Design review of the part shown in the three views and the two pictorial views. Dimensions are in mm from the part's minimum x, y and z. A direction names the side the tool comes from. Coordinates: 2 decimals unless noted, no trailing zeros. Loops run counter-clockwise (first coordinate to the right, second up) from the corner with the lowest first, then second, coordinate; pieces in that order, holes last. Notation, with made-up numbers: (12, 78.5) - (24, 78.5) arc R19 ccw to (24, 104.5) - close; hole circle Ø2 at (53.5, 46). An arc over 180 degrees is marked (long way). One line per item, written item: value. Start each with the question number.
1. Take a section at A-A, the plane x = 5.5. State the section outline as (y, z) points, and give its area (3 significant figures).
2. Take a section at D-D, the plane x = 1.75. State the section outline as (y, z) points.
3. To check wall thickness, follow line 1 (X direction, y = 2.1, z = 3.75); line 2 (X direction, y = 0.65, z = 6) (1 decimal). State the ranges of each line that lie inside material, in increasing order. Write a range as from..to.
4. Take a section at C-C, the plane z = 1.25. State the section outline as (x, y) points.
5. Take a section at B-B, the plane y = 2. State the section outline as (x, z) points.
6. Insertion check: pin 1 (5 mm diameter, centred on x = 2.5, z = 4, fed in from +Y); pin 2 (1.5 mm diameter, centred on x = 3.5, z = 7, fed in from +Y). Each pin has a flat end and moves straight along its axis. Give the tip position at first contact, or say it passes through.
7. For the marked faces 1, 2, 3, 4 and 5, list the 3-axis set-ups (+Z, -Z, +X, -X, +Y, -Y) from which the entire face can be reached by the end or side of a thin tool; tool diameter is ignored.
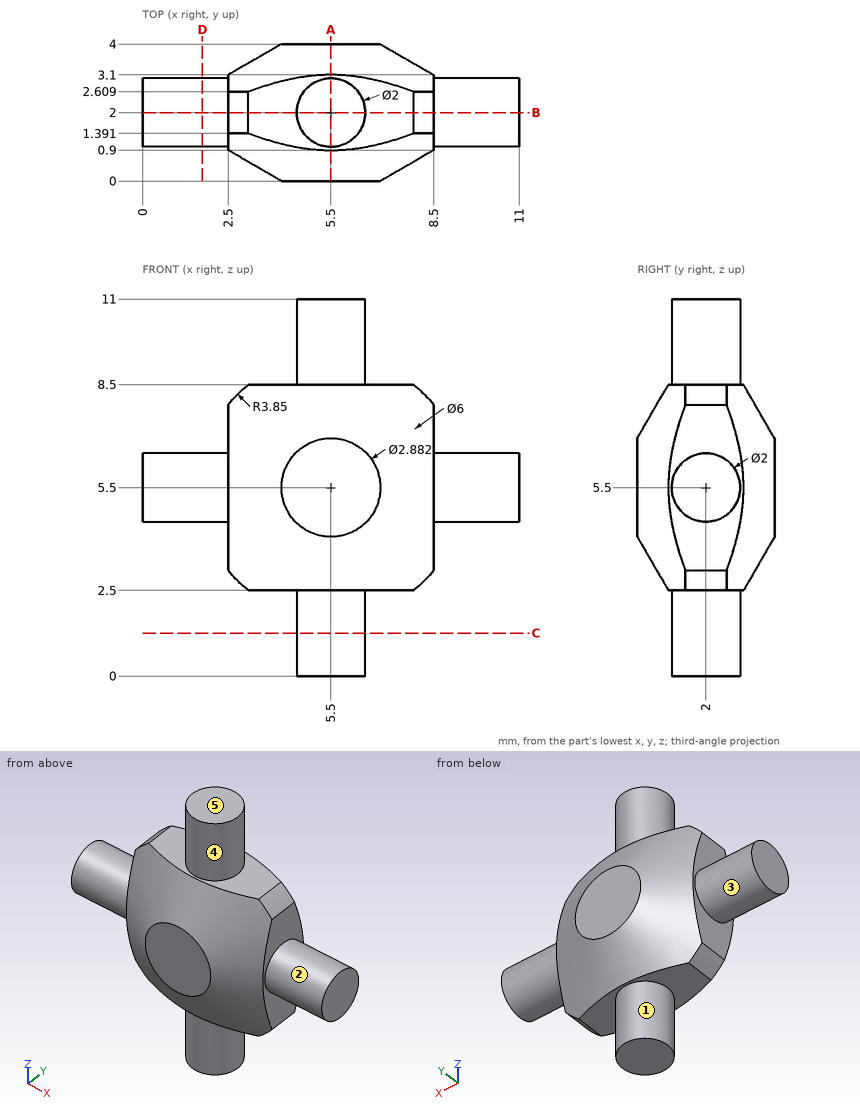
Solutions:
1. outline: (0, 4.06) - (0.9, 2.5) - (1, 2.5) - (1, 0) - (3, 0) - (3, 2.5) - (3.1, 2.5) - (4, 4.06) - (4, 6.94) - (3.1, 8.5) - (3, 8.5) - (3, 11) - (1, 11) - (1, 8.5) - (0.9, 8.5) - (0, 6.94) - close
1. area: 31.2 mm2
2. outline: circle Ø2 at (2, 5.5)
3. line 1: 2.5..8.5
3. line 2: 3..8
4. outline: circle Ø2 at (5.5, 2)
5. outline: (0, 4.5) - (2.5, 4.5) - (2.5, 3.09) arc R3.85 ccw to (3.09, 2.5) - (4.5, 2.5) - (4.5, 0) - (6.5, 0) - (6.5, 2.5) - (7.91, 2.5) arc R3.85 ccw to (8.5, 3.09) - (8.5, 4.5) - (11, 4.5) - (11, 6.5) - (8.5, 6.5) - (8.5, 7.91) arc R3.85 ccw to (7.91, 8.5) - (6.5, 8.5) - (6.5, 11) - (4.5, 11) - (4.5, 8.5) - (3.09, 8.5) arc R3.85 ccw to (2.5, 7.91) - (2.5, 6.5) - (0, 6.5) - close
6. pin 1: y = 4
6. pin 2: y = 3.82
7. face 1: -Z
7. face 2: +X
7. face 3: -X
7. face 4: +Z
7. face 5: +Z, +X, -X, +Y, -Y
